Could you check a few things on this model? Use its own coordinates, in mm. Face numbers are marked on the shaded views. A direction names the side the tool comes from. Round coordinates to 2 decimals unless told otherwise and drop trailing zeros. Write each loop counter-clockwise with the first axis right and the second up, starting at its lowest first coordinate (ties: lowest second). Pieces come first, ordered by that corner, then holes. Notation, with made-up numbers: (21, -10) - (69, -10) arc R34 cw to (69, 22) - close; hole circle Ø3 at (-10.5, 58). An arc over 180 degrees is marked (long way). Put each result on its own line as item: value.
from build123d import *

# Parameters (mm, degrees)
SKETCH1_R           = 22
SKETCH1_W           = 4
SKETCH1_H           = 4.8
BOSS_EXTRUDE1_DEPTH = 5
BOSS_EXTRUDE2_DEPTH = 5
SKETCH3_R           = 5
CUT_EXTRUDE1_DEPTH  = 2.5


with BuildPart() as part:
    # Sketch1 → Boss-Extrude1 (new body)
    with BuildSketch(Plane(origin=(0, 0, 0), x_dir=(1, 0, 0), z_dir=(0, 1, 0))):
        Circle(SKETCH1_R)
        with Locations((-23.868699093, 0)):
            Rectangle(SKETCH1_W, SKETCH1_H)
        with BuildLine():
            Line((21.868699093, 2.4), (25.135681809, 2.4))
            ThreePointArc((25.135681809, 2.4), (24.45754678, 6.276217454), (23.185394109, 10))
            Line((23.185394109, 10), (25.935394109, 10))
            ThreePointArc((25.935394109, 10), (27.796486605, 0), (25.935394109, -10))
            Line((25.935394109, -10), (23.185394109, -10))
            ThreePointArc((23.185394109, -10), (24.45754678, -6.276217454), (25.135681809, -2.4))
            Line((25.135681809, -2.4), (21.868699093, -2.4))
            Line((21.868699093, -2.4), (21.868699093, 2.4))
        make_face()
    extrude(amount=BOSS_EXTRUDE1_DEPTH)

    # Sketch2 → Boss-Extrude2 (add)
    with BuildSketch(Plane(origin=(0, 5, 0), x_dir=(1, 0, 0), z_dir=(0, 1, 0))):
        with BuildLine():
            Line((-29.110423057, 12), (-22.216266563, 12))
            ThreePointArc((-22.216266563, 12), (-25.131713885, 2.441199952), (-24.110423057, -7.5))
            Line((-24.110423057, -7.5), (-29.110423057, -7.5))
            Line((-29.110423057, -7.5), (-29.110423057, 12))
        make_face()
    extrude(amount=-BOSS_EXTRUDE2_DEPTH)

    # Sketch3 → Cut-Extrude1 (cut)
    with BuildSketch(Plane(origin=(0, 5, 0), x_dir=(1, 0, 0), z_dir=(0, 1, 0))):
        Circle(SKETCH3_R)
    extrude(amount=-CUT_EXTRUDE1_DEPTH, mode=Mode.SUBTRACT)


solid = part.part
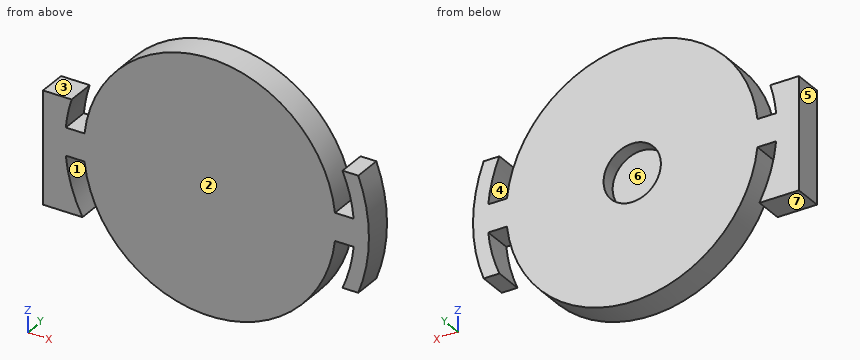
(1) I'm going to push flat-ended pins straight in: pin 1 (1.6 mm diameter, centred on x = 24.5, y = 2, fed in from -Z); pin 2 (2.5 mm diameter, centred on x = -26, y = 2, fed in from +Z); pin 3 (1.5 mm diameter, centred on y = 4.5, z = -5, fed in from +X). Where does each tip first touch, or does it pass through?
Values found:
pin 1: stops at z = -10
pin 2: stops at z = 7.5
pin 3: stops at x = 27.47
(2) Please list where these lines run through material, in increasing order: probe 1 along Z at (x, y) = (0, 3.45); probe 2 along X at (y, z) = (3.95, 0); probe 3 along X at (y, z) = (4, -8). Write a range as from..to.
Values found:
probe 1: z = -22..-5, 5..22
probe 2: x = -29.11..-5, 5..27.8
probe 3: x = -29.11..-23.95, -20.49..20.49, 23.95..26.62
(3) Imagine slicing it at B-B, the plane y = 3.6. List the corners of the cut face in (x, z) for me.
Values found:
outline: (-29.11, -12) - (-22.22, -12) arc R25.25 cw to (-25.14, -2.4) - (-21.87, -2.4) arc R22 ccw to (21.87, -2.4) - (25.14, -2.4) arc R25.25 cw to (23.19, -10) - (25.94, -10) arc R27.8 ccw to (25.94, 10) - (23.19, 10) arc R25.25 cw to (25.14, 2.4) - (21.87, 2.4) arc R22 ccw to (-21.87, 2.4) - (-25.14, 2.4) arc R25.25 cw to (-24.11, 7.5) - (-29.11, 7.5) - close; hole circle Ø10 at (0, 0)
(4) If we mould it in two halves opening along Z, with no side actions, what happens to the marked faces 1, 2, 3 and 4? For each: pulls with the +Z half, pulls with the -Z half, needs draft (parallel to the pull), parting line crosses it, or undercut.
Values found:
face 1: undercut
face 2: needs draft
face 3: pulls with the +Z half
face 4: undercut
(5) Imagine slicing it at A-A, the plane x = -23.5. List the corners of the cut face in (y, z) for me, then the cut area to 3 significant figures.
Values found:
outline: (0, -12) - (5, -12) - (5, -9.24) - (0, -9.24) - close; (0, -2.4) - (5, -2.4) - (5, 2.4) - (0, 2.4) - close
area: 37.8 mm^2
(6) For the marked faces 5, 6 and 7, which set-ups out of +Z, -Z, +X, -X, +Y, -Y let a thin tool reach every point of the face, with its end or its side?
Values found:
face 5: +Z, -Z, -X, +Y, -Y
face 6: +Y
face 7: -Z, -X, +Y, -Y
(7) Imagine slicing it at D-D, the plane x = 0. List the corners of the cut face in (y, z) for me, then the cut area to 3 significant figures.
Values found:
outline: (0, -22) - (5, -22) - (5, -5) - (2.5, -5) - (2.5, 5) - (5, 5) - (5, 22) - (0, 22) - close
area: 195 mm^2
(8) Imagine slicing it at C-C, the plane z = 0. List the corners of the cut face in (x, y) for me, then the cut area to 3 significant figures.
Values found:
outline: (-29.11, 0) - (27.8, 0) - (27.8, 5) - (5, 5) - (5, 2.5) - (-5, 2.5) - (-5, 5) - (-29.11, 5) - close
area: 260 mm^2
